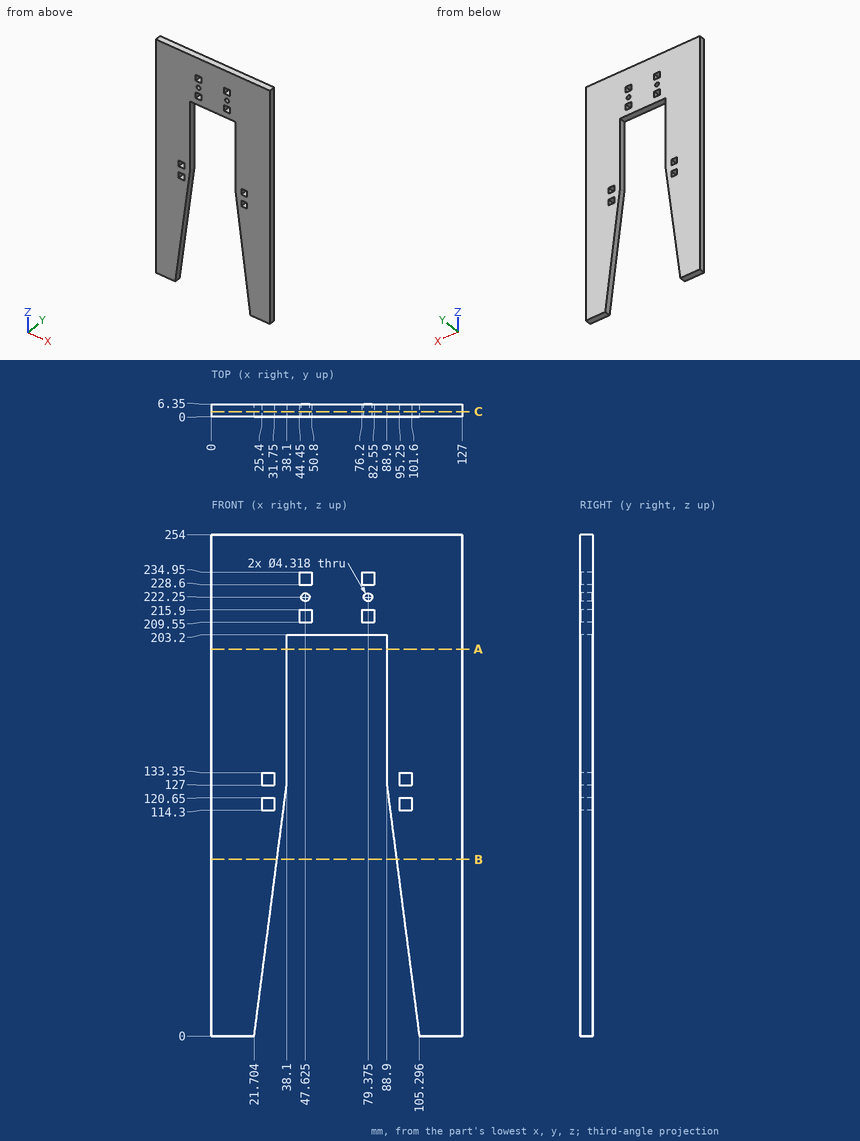
Part print with two shaded views. Sizes in mm from the minimum x, y, z corner. Round coordinates to 2 decimals unless told otherwise and drop trailing zeros. Write each loop counter-clockwise with the first axis right and the second up, starting at its lowest first coordinate (ties: lowest second). Pieces come first, ordered by that corner, then holes. Notation, with made-up numbers: (23, -4) -> (62, -4) arc R22 ccw to (62, 35) -> close; hole circle Ø2 at (15.5, -15.75). An arc over 180 degrees is marked (long way). Put each result on its own line as item: value.
Item 1: Slice it at B-B, the plane z = 89.5. Give the cut face in (x, y).
Here are the results:
outline: (0, 0) -> (33.26, 0) -> (33.26, 6.35) -> (0, 6.35) -> close; (93.74, 0) -> (127, 0) -> (127, 6.35) -> (93.74, 6.35) -> close
Item 2: Wall check: probe 1 along X at (y, z) = (5, 222.25); probe 2 along Z at (x, y) = (82, 0.75); probe 3 along X at (y, z) = (2.5, 148). Give the ranges that are in metal, low to high. Write a range as from..to.
Here are the results:
probe 1: x = 0..45.47, 49.78..77.22, 81.53..127
probe 2: z = 203.2..209.55, 215.9..228.6, 234.95..254
probe 3: x = 0..38.1, 88.9..127
Item 3: Slice it at A-A, the plane z = 196. Give the cut face in (x, y).
Here are the results:
outline: (0, 0) -> (38.1, 0) -> (38.1, 6.35) -> (0, 6.35) -> close; (88.9, 0) -> (127, 0) -> (127, 6.35) -> (88.9, 6.35) -> close
Item 4: Slice it at C-C, the plane y = 2.5. Count the separate pieces of the cut face and the enclosed holes in it, plus the area to 3 significant figures.
Here are the results:
separate pieces: 1
enclosed holes: 10
area: 19,500 mm^2
Item 5: Flat gauge pins, fed straight in: P1, Ø5.5, axis at x = 47.625, z = 222.25, coming from the -Y side; P2, Ø3, axis at x = 80.5, y = 4.5, coming from the -Z side. Where does each tip first touch, or does it go through?
Here are the results:
P1: stops at y = 0
P2: stops at z = 203.2
